```python
from build123d import *

# Parameters (mm, degrees)
SKETCH1_W           = 38.1
SKETCH1_H           = 38.1
SKETCH1_R           = 4
SKETCH1_R_2         = 1.5875
SKETCH1_R_3         = 1.25
BOSS_EXTRUDE1_DEPTH = 3.175
SKETCH4_R           = 1.7272
CUT_EXTRUDE2_DEPTH  = 10.795
SKETCH7_R           = 2.15265
CUT_EXTRUDE3_DEPTH  = 7.3500001
CIRPATTERN1_COUNT   = 4
SKETCH6_W           = 38.1
SKETCH6_H           = 38.1
SKETCH6_R           = 6.5
SKETCH6_R_2         = 2.15265
BOSS_EXTRUDE2_DEPTH = 3.175
FILLET1_R           = 2.54
FILLET2_R           = 2.54
SKETCH8_R           = 3.96875
SKETCH8_R_2         = 2.3876
BOSS_EXTRUDE3_DEPTH = 3.937
CIRPATTERN2_COUNT   = 4


with BuildPart() as part:
    # Sketch1 → Boss-Extrude1 (new body, symmetric)
    with BuildSketch(Plane(origin=(0, 0, 0), x_dir=(1, 0, 0), z_dir=(0, 1, 0))):
        Rectangle(SKETCH1_W, SKETCH1_H)
        Circle(SKETCH1_R, mode=Mode.SUBTRACT)
        with Locations((8.838834765, 8.838834765)):
            Circle(SKETCH1_R_2, mode=Mode.SUBTRACT)
        with Locations((8.838834765, -8.838834765)):
            Circle(SKETCH1_R_2, mode=Mode.SUBTRACT)
        with Locations((-8.838834765, -8.838834765)):
            Circle(SKETCH1_R_2, mode=Mode.SUBTRACT)
        with Locations((-8.838834765, 8.838834765)):
            Circle(SKETCH1_R_2, mode=Mode.SUBTRACT)
        with Locations((-14.5, 0)):
            Circle(SKETCH1_R_3, mode=Mode.SUBTRACT)
        with Locations((0, 14.5)):
            Circle(SKETCH1_R_3, mode=Mode.SUBTRACT)
        with Locations((14.5, 0)):
            Circle(SKETCH1_R_3, mode=Mode.SUBTRACT)
        with Locations((0, -14.5)):
            Circle(SKETCH1_R_3, mode=Mode.SUBTRACT)
    extrude(amount=BOSS_EXTRUDE1_DEPTH, both=True)

    # Sketch4 → Cut-Extrude2 (cut)
    with BuildSketch(Plane.XY.offset(19.05)):
        with Locations((-5.55625, 0)):
            Circle(SKETCH4_R)
        with Locations((5.55625, 0)):
            Circle(SKETCH4_R)
    cut_extrude2 = extrude(amount=-CUT_EXTRUDE2_DEPTH, mode=Mode.SUBTRACT)

    # Sketch7 → Cut-Extrude3 (cut, through all)
    with BuildSketch(Plane.XZ.offset(3.175)):
        with Locations((-15.08125, 15.08125)):
            Circle(SKETCH7_R)
        with Locations((15.08125, 15.08125)):
            Circle(SKETCH7_R)
        with Locations((15.08125, -15.08125)):
            Circle(SKETCH7_R)
        with Locations((-15.08125, -15.08125)):
            Circle(SKETCH7_R)
    extrude(amount=-CUT_EXTRUDE3_DEPTH, mode=Mode.SUBTRACT)

    # CirPattern1: Cut-Extrude2 ×4 about axis
    cirpattern1_axis = Axis((0, 0, 0), (0, 1, 0))
    for i in range(1, CIRPATTERN1_COUNT):
        add(cut_extrude2.rotate(cirpattern1_axis, i * 360 / CIRPATTERN1_COUNT), mode=Mode.SUBTRACT)

    # Fillet1
    fillet1_edges = [part.edges().sort_by_distance(p)[0] for p in [
        (19.05, 0, 19.05),
        (-19.05, 0, 19.05),
        (-19.05, 0, -19.05),
        (19.05, 0, -19.05),
    ]]
    fillet(fillet1_edges, radius=FILLET1_R)


with BuildPart() as body_2:
    # Sketch6 → Boss-Extrude2 (new body)
    with BuildSketch(Plane(origin=(0, -32.512, 0), x_dir=(-1, 0, 0), z_dir=(0, -1, 0))):
        Rectangle(SKETCH6_W, SKETCH6_H)
        Circle(SKETCH6_R, mode=Mode.SUBTRACT)
        with Locations((-15.08125, 15.08125)):
            Circle(SKETCH6_R_2, mode=Mode.SUBTRACT)
        with Locations((15.08125, 15.08125)):
            Circle(SKETCH6_R_2, mode=Mode.SUBTRACT)
        with Locations((15.08125, -15.08125)):
            Circle(SKETCH6_R_2, mode=Mode.SUBTRACT)
        with Locations((-15.08125, -15.08125)):
            Circle(SKETCH6_R_2, mode=Mode.SUBTRACT)
    extrude(amount=BOSS_EXTRUDE2_DEPTH)

    # Fillet2
    fillet2_edges = [body_2.edges().sort_by_distance(p)[0] for p in [
        (-19.05, -34.0995, 19.05),
        (19.05, -34.0995, 19.05),
        (19.05, -34.0995, -19.05),
        (-19.05, -34.0995, -19.05),
    ]]
    fillet(fillet2_edges, radius=FILLET2_R)


with BuildPart() as body_3:
    # Sketch8 → Boss-Extrude3 (new body)
    with BuildSketch(Plane(origin=(0, -32.512, 0), x_dir=(1, 0, 0), z_dir=(0, 1, 0))):
        with Locations((-15.08125, 15.08125)):
            Circle(SKETCH8_R)
        with Locations((-15.08125, 15.08125)):
            Circle(SKETCH8_R_2, mode=Mode.SUBTRACT)
    extrude(amount=BOSS_EXTRUDE3_DEPTH)


with BuildPart() as cirpattern2_1:
    # CirPattern2: pattern copy
    add(body_3.part.rotate(Axis((0, 0, 0), (0, 1, 0)), 1 * 360 / CIRPATTERN2_COUNT))


with BuildPart() as cirpattern2_2:
    # CirPattern2: pattern copy
    add(body_3.part.rotate(Axis((0, 0, 0), (0, 1, 0)), 2 * 360 / CIRPATTERN2_COUNT))


with BuildPart() as cirpattern2_3:
    # CirPattern2: pattern copy
    add(body_3.part.rotate(Axis((0, 0, 0), (0, 1, 0)), 3 * 360 / CIRPATTERN2_COUNT))


solid = cirpattern2_3.part
```
Geometry check sheet. Reference: the model listing, model coordinates, mm. Give positions to 0.01 mm unless a question says otherwise; leave off trailing zeros. Write each loop counter-clockwise with the first axis right and the second up, starting at its lowest first coordinate (ties: lowest second). Pieces come first, ordered by that corner, then holes.
1) Material ranges on L1, parallel to Z at x = 15.25, y = -31.65; L2, parallel to Z at x = 13.5, y = -30.8; L3, parallel to X at y = -30.9, z = -14, recorded low to high.
2) Section check B-B, the plane x = 13.75. Record the boundary of the cut face in (y, z) (3 decimals), and give its area (3 significant figures).
3) Section check D-D, the plane z = -17.75. Record the boundary of the cut face in (x, y) (3 decimals).
4) Release check for a two-part mould opening along X. For faces 1 (the cylindrical face through (17.094, -30.571, -13.798)), 2 (the flat face through (13, -28.575, -13)), 3 (the cylindrical face through (11.56, -30.57, -13.25)) record: pulls with the +X half, pulls with the -X half, needs draft (parallel to the pull), parting line crosses it, or undercut.
5) Gauge pin test, flat ends, axial feed: pin 1 (1 mm diameter, centred on y = -30.5, z = -16.5, fed in from -X); pin 2 (1 mm diameter, centred on y = -31.5, z = -13, fed in from +X). Record the tip position at first contact, or that the pin passes through.
6) Section check A-A, the plane z = -13.25. Record the boundary of the cut face in (x, y) (3 decimals), and give its area (3 significant figures).
7) Section check C-C, the plane y = -30. Record the boundary of the cut face in (x, z), and give its area (3 significant figures).
Computed:
1. L1: z = -19.05 to -17.46, -12.7 to -11.12
1. L2: z = -18.72 to -16.87, -13.29 to -11.44
1. L3: x = 11.26 to 12.95, 17.21 to 18.9
2. outline: (-32.512, -18.82) - (-28.575, -18.82) - (-28.575, -17.063) - (-32.512, -17.063) - close; (-32.512, -13.099) - (-28.575, -13.099) - (-28.575, -11.342) - (-32.512, -11.342) - close
2. area: 13.8 mm2
3. outline: (12.144, -32.512) - (18.019, -32.512) - (18.019, -28.575) - (12.144, -28.575) - close
4. face 1: undercut
4. face 2: needs draft
4. face 3: parting line crosses it
5. pin 1: stops at x = 11.22
5. pin 2: stops at x = 18.72
6. outline: (11.56, -32.512) - (13.549, -32.512) - (13.549, -28.575) - (11.56, -28.575) - close; (16.613, -32.512) - (18.602, -32.512) - (18.602, -28.575) - (16.613, -28.575) - close
6. area: 15.7 mm2
7. outline: circle Ø7.94 at (15.08, -15.08); hole circle Ø4.78 at (15.08, -15.08)
7. area: 31.6 mm2
